from build123d import *

# Parameters (mm, degrees)
F0_W      = 15
F0_H      = 21
F1_DEPTH  = 1.25
F2_W      = 15
F2_H      = 6
F2_H_2    = 3
F3_DEPTH  = 20
F4_W      = 3
F4_H      = 15
F5_DEPTH  = 20
F6_R      = 2.505
F7_DEPTH  = 25
F8_R      = 2.505
F9_DEPTH  = 25
F10_SIZE  = 2
F11_DEPTH = 3
F12_SIZE  = 2.7
F13_SIZE  = 1


with BuildPart() as f1:
    # F0 (on Top) → F1 (new body, symmetric)
    with BuildSketch(Plane.XY):
        Rectangle(F0_W, F0_H)
    extrude(amount=F1_DEPTH, both=True)

    # F2 (on face) → F3 (join)
    with BuildSketch(Plane.XY.offset(1.25)):
        with Locations((0, -7.5)):
            Rectangle(F2_W, F2_H)
        Rectangle(F2_W, F2_H_2)
        with Locations((0, 7.5)):
            Rectangle(F2_W, F2_H)
    extrude(amount=F3_DEPTH)

    # F4 (on face) → F5 (join)
    with BuildSketch(Plane(origin=(0, 0, -1.25), x_dir=(1, 0, 0), z_dir=(0, 0, -1))):
        with Locations((-3, 0)):
            Rectangle(F4_W, F4_H)
        with Locations((3, 0)):
            Rectangle(F4_W, F4_H)
    extrude(amount=F5_DEPTH)

    # F6 (on face) → F7 (cut)
    with BuildSketch(Plane.XZ.offset(10.5)):
        with BuildLine():
            ThreePointArc((0, 21.25), (5.3033008589, 19.0533008589), (7.5, 13.75))
            Line((7.5, 13.75), (7.5, 21.25))
            Line((7.5, 21.25), (0, 21.25))
        make_face()
        with BuildLine():
            ThreePointArc((-7.5, 13.75), (-5.3033008589, 19.0533008589), (0, 21.25))
            Line((0, 21.25), (-7.5, 21.25))
            Line((-7.5, 21.25), (-7.5, 13.75))
        make_face()
        with Locations((0, 13.75)):
            Circle(F6_R)
    extrude(amount=-F7_DEPTH, mode=Mode.SUBTRACT)

    # F8 (on face) → F9 (cut)
    with BuildSketch(Plane(origin=(-4.5, 0, 0), x_dir=(0, -1, 0), z_dir=(-1, 0, 0))):
        with BuildLine():
            Line((7.5, -21.25), (7.5, -13.75))
            ThreePointArc((7.5, -13.75), (5.3033008589, -19.0533008589), (0, -21.25))
            Line((0, -21.25), (7.5, -21.25))
        make_face()
        with BuildLine():
            ThreePointArc((0, -21.25), (-5.3033008589, -19.0533008589), (-7.5, -13.75))
            Line((-7.5, -13.75), (-7.5, -21.25))
            Line((-7.5, -21.25), (0, -21.25))
        make_face()
        with Locations((0, -13.75)):
            Circle(F8_R)
    extrude(amount=-F9_DEPTH, mode=Mode.SUBTRACT)

    # F10
    f10_edges = [f1.edges().sort_by_distance(p)[0] for p in [
        (-7.5, 0, -1.25),
        (0, 10.5, -1.25),
        (0, -10.5, -1.25),
        (7.5, 0, -1.25),
    ]]
    chamfer(f10_edges, length=F10_SIZE)

    # F6 (on face) → F11 (cut)
    with BuildSketch(Plane.XZ.offset(10.5)):
        Polygon((4.0080889509, 16.0684814631), (-0.0038193698, 18.3803475837), (-4.0119083207, 16.0618661206), (-4.0080889509, 11.4315185369), (0.0038193698, 9.1196524163), (4.0119083207, 11.4381338794), align=None)
        with Locations((0, 13.75)):
            Circle(F6_R, mode=Mode.SUBTRACT)
    extrude(amount=-F11_DEPTH, mode=Mode.SUBTRACT)

    # F12
    f12_edges = [f1.edges().sort_by_distance(p)[0] for p in [
        (-2.505, 10.5, 13.75),
    ]]
    chamfer(f12_edges, length=F12_SIZE)

    # F13
    f13_edges = [f1.edges().sort_by_distance(p)[0] for p in [
        (0, 10.5, 21.25),
        (7.5, 10.5, 7.25),
        (-7.5, 10.5, 7.25),
        (7.5, -10.5, 7.25),
        (-7.5, -10.5, 7.25),
        (0, -10.5, 21.25),
    ]]
    chamfer(f13_edges, length=F13_SIZE)


solid = f1.part
Read the model definition and answer for the solid it produces. Units are mm, in the model's axes. A direction names the side the tool comes from. Round coordinates to 2 decimals unless told otherwise and drop trailing zeros. Order: outer loops, then holes, each group sorted by start corner. A loop starts at its lowest first (then second) coordinate and runs counter-clockwise, first axis right, second up.
1) For faces 4 (the face through (-3, 7.5, -7)), 5 (the face through (-3, -7.5, -7)), 6 (the face through (-4.5, 0, -11)), 7 (the face through (0, -3, 1.25)), determine the directions among +Z, -Z, +X, -X, +Y, -Y from which every point of the face is accessible in a straight line to the end or side of a thin tool.
2) The mould has two halves that part along X. Classify faces 1 (the face through (1.16, -0.02, 11.53)), 2 (the face through (0, 4.5, 11)), 3 (the face through (-7, -10, 7)): released by +X, released by -X, zero draft, split by the parting line, or undercut.
3) Straight lines are drawn through the part: L1, parallel to Y at x = 5.5, z = 16; L2, parallel to X at y = 6.5, z = -10; L3, parallel to Y at x = -1.5, z = 17. For each, find the intervals that lie inside material, in ascending order.
4) The part is cut by section B-B on y = -8. Write down the section's boundary in (x, z), plus the area to 3 significant figures.
5) The part is cut by section C-C on z = -4. Write down the section's boundary in (x, y), plus the area to 3 significant figures.
6) Flat-ended cylindrical pins translate along their axes: pin 1 (1.5 mm diameter, centred on x = -2.5, z = -7, fed in from -Y); pin 2 (1 mm diameter, centred on x = -3, y = 0.5, fed in from +Z); pin 3 (5 mm diameter, centred on y = -8, z = -11.5, fed in from +X). Find the tip coordinate at first contact, or state that the pin passes through.
7) The part is cut by section D-D on x = 2. Give the number of separate pieces and of enclosed holes in the cut face, plus the area to 3 significant figures.
8) The part is cut by section A-A on y = 0. Write down the section's boundary in (x, z) (3 decimals).
Resolved:
1. face 4: -Z, +X, -X, +Y
1. face 5: -Z, +X, -X, -Y
1. face 6: -Z, -X, +Y, -Y
1. face 7: +Z, +X, -X
2. face 1: undercut
2. face 2: zero draft
2. face 3: released by -X
3. L1: y = -10.5 to -4.5, -1.5 to 1.5, 4.5 to 10.5
3. L2: x = -4.5 to -1.5, 1.5 to 4.5
3. L3: y = -7.5 to -4.5, -1.5 to 1.5, 4.5 to 8.87
4. outline: (-7.5, 0.75) - (-5.5, -1.25) - (5.5, -1.25) - (7.5, 0.75) - (7.5, 13.75) arc R7.5 ccw to (-7.5, 13.75) - close; hole (-4.01, 11.43) - (0, 9.12) - (4.01, 11.44) - (4.01, 16.07) - (0, 18.38) - (-4.01, 16.06) - close
4. area: 254 mm2
5. outline: (-4.5, -7.5) - (-1.5, -7.5) - (-1.5, 7.5) - (-4.5, 7.5) - close; (1.5, -7.5) - (4.5, -7.5) - (4.5, 7.5) - (1.5, 7.5) - close
5. area: 90.0 mm2
6. pin 1: stops at y = -7.5
6. pin 2: stops at z = 20.82
6. pin 3: stops at x = 4.5
7. separate pieces: 4
7. enclosed holes: 1
7. area: 533 mm2
8. outline: (-7.5, 0.75) - (-5.5, -1.25) - (-4.5, -1.25) - (-4.5, -11.245) - (-1.5, -11.245) - (-1.5, -1.25) - (1.5, -1.25) - (1.5, -11.245) - (4.5, -11.245) - (4.5, -1.25) - (5.5, -1.25) - (7.5, 0.75) - (7.5, 13.75) arc R7.5 ccw to (-7.5, 13.75) - close; (-4.5, -21.25) - (-1.5, -21.25) - (-1.5, -16.255) - (-4.5, -16.255) - close; (1.5, -21.25) - (4.5, -21.25) - (4.5, -16.255) - (1.5, -16.255) - close; hole circle Ø5.01 at (0, 13.75)
